Could you check a few things on this model? Use its own coordinates, in mm. A direction names the side the tool comes from. Coordinates: 2 decimals unless noted, no trailing zeros. Loops run counter-clockwise (first coordinate to the right, second up) from the corner with the lowest first, then second, coordinate; pieces in that order, holes last.
1) Thinking about a two-plate mould opening in Z: for faces 5 (the face through (6.4, 145, -75)), 6 (the face through (3, 102, -52.4)), 7 (the face through (3, -3, -2.7)), which applies, released by +Z, released by -Z, zero draft, split by the parting line, or undercut?
2) Imagine slicing it at A-A on y = 20. Please give me the cut outline in (x, z), plus the area to 3 significant figures.
3) Imagine slicing it at C-C on y = 118. Please give me the cut outline in (x, z), plus the area to 3 significant figures.
4) Imagine slicing it at D-D on z = -10. Please give me the cut outline in (x, y), plus the area to 3 significant figures.
5) Will these pins go through, and if not, where does the flat tip stop? P1, Ø1.9, axis at x = 3.5, z = -75.5, coming from the -Y side; P2, Ø3.5, axis at y = 264, z = -76.2, coming from the -X side; P3, Ø1.9, axis at x = 4.5, y = 74.5, coming from the +Z side.
6) For faces 1 (the face through (3, 0, -49)), 2 (the face through (3, 291, -43.7)), 3 (the face through (3, 75, -52.4)), 4 (the face through (3, -6.4, -117)), which set-ups out of +Z, -Z, +X, -X, +Y, -Y let a thin tool reach every point of the face, with its end or its side?
7) If I drill on line 1 along Z through (x, y) = (3.5, 288) (3 decimals); line 2 along Z through (x, y) = (3.75, 20); line 3 along Z through (x, y) = (6, 107.5), over which ranges is the centre line in solid material (lowest first)?
8) Imagine slicing it at B-B on x = 4.5. Give the number of separate pieces and of enclosed holes in the cut face, plus the area to 3 significant figures.
Autodesk Inventor part; units mm, degrees
ref_plane "YZ Plane" through (0, 0, 0) normal (1, 0, 0) x (0, 1, 0)
ref_plane "XZ Plane" through (0, 0, 0) normal (0, 1, 0) x (-1, 0, 0)
ref_plane "XY Plane" through (0, 0, 0) normal (0, 0, 1) x (1, 0, 0)
sketch "Sketch1" plane through (0, 0, 0) normal (1, 0, 0) x (0, 1, 0)
  line L0 (0, 0) -> (0, -152.4) construction
  line L1 (390, -43.7) -> (0, -43.7) construction
  line L2 (0, -43.7) -> (0, -108.7) construction
  line L3 (0, -108.7) -> (390, -108.7) construction
  line L4 (390, -108.7) -> (390, -43.7) construction
  line L5 (0, 0) -> (0, -152.4)
  line L6 (0, 0) -> (195, -43.7)
  line L7 (0, -152.4) -> (195, -108.7)
  line L8 (195, -43.7) -> (390, -43.7)
  line L9 (390, -43.7) -> (390, -108.7)
  line L10 (390, -108.7) -> (195, -108.7)
  circle A0 centre (384, -76.2) radius 2.875
  line L11 (390, -66.2) -> (366, -66.2)
  line L12 (366, -86.2) -> (390, -86.2)
  line L13 (390, -86.2) -> (390, -66.2)
  circle A1 centre (372, -76.2) radius 2.875
  line L14 (0, -2.7) -> (-6.4, -2.7)
  line L15 (-6.4, -2.7) -> (-6.4, -14.7)
  line L16 (-6.4, -14.7) -> (0, -14.7)
  line L17 (0, -14.7) -> (0, -2.7)
  line L18 (-6.4, -29.7) -> (-6.4, -41.7)
  line L19 (-6.4, -41.7) -> (0, -41.7)
  line L20 (0, -29.7) -> (-6.4, -29.7)
  line L21 (-6.4, -56.7) -> (-6.4, -68.7)
  line L22 (-6.4, -68.7) -> (0, -68.7)
  line L23 (0, -56.7) -> (-6.4, -56.7)
  line L24 (-6.4, -83.7) -> (-6.4, -95.7)
  line L25 (-6.4, -95.7) -> (0, -95.7)
  line L26 (0, -83.7) -> (-6.4, -83.7)
  line L27 (-6.4, -110.7) -> (-6.4, -122.7)
  line L28 (-6.4, -122.7) -> (0, -122.7)
  line L29 (0, -110.7) -> (-6.4, -110.7)
  line L30 (-6.4, -137.7) -> (-6.4, -149.7)
  line L31 (-6.4, -149.7) -> (0, -149.7)
  line L32 (0, -137.7) -> (-6.4, -137.7)
  line L33 (27, -46) -> (15, -46)
  line L34 (15, -46) -> (15, -52.4)
  line L35 (15, -52.4) -> (27, -52.4)
  line L36 (27, -52.4) -> (27, -46)
  line L37 (27, -49.2) -> (15, -49.2) construction
  line L38 (42, -52.4) -> (54, -52.4)
  line L39 (54, -46) -> (42, -46)
  line L40 (42, -46) -> (42, -52.4)
  line L41 (54, -52.4) -> (54, -46)
  line L42 (69, -52.4) -> (81, -52.4)
  line L43 (81, -46) -> (69, -46)
  line L44 (69, -46) -> (69, -52.4)
  line L45 (81, -52.4) -> (81, -46)
  line L46 (96, -52.4) -> (108, -52.4)
  line L47 (108, -46) -> (96, -46)
  line L48 (96, -46) -> (96, -52.4)
  line L49 (108, -52.4) -> (108, -46)
  line L50 (96, -106.4) -> (108, -106.4)
  line L51 (108, -100) -> (96, -100)
  line L52 (96, -100) -> (96, -106.4)
  line L53 (108, -106.4) -> (108, -100)
  line L54 (69, -106.4) -> (81, -106.4)
  line L55 (69, -100) -> (69, -106.4)
  line L56 (81, -100) -> (69, -100)
  line L57 (81, -106.4) -> (81, -100)
  line L58 (42, -106.4) -> (54, -106.4)
  line L59 (54, -100) -> (42, -100)
  line L60 (54, -106.4) -> (54, -100)
  line L61 (42, -100) -> (42, -106.4)
  line L62 (15, -106.4) -> (27, -106.4)
  line L63 (15, -100) -> (15, -106.4)
  line L64 (27, -100) -> (15, -100)
  line L65 (27, -106.4) -> (27, -100)
  line L66 (366, -66.2) -> (366, -86.2)
  circle A2 centre (360, -76.2) radius 2.875
  circle A3 centre (348, -76.2) radius 2.875
  line L67 (366, -66.2) -> (342, -66.2)
  line L68 (342, -86.2) -> (366, -86.2)
  line L69 (342, -66.2) -> (342, -86.2)
  circle A4 centre (336, -76.2) radius 2.875
  circle A5 centre (324, -76.2) radius 2.875
  line L70 (342, -66.2) -> (318, -66.2)
  line L71 (318, -86.2) -> (342, -86.2)
  line L72 (318, -66.2) -> (318, -86.2)
  circle A6 centre (312, -76.2) radius 2.875
  circle A7 centre (300, -76.2) radius 2.875
  line L73 (318, -66.2) -> (294, -66.2)
  line L74 (294, -86.2) -> (318, -86.2)
  line L75 (294, -66.2) -> (294, -86.2)
  circle A8 centre (288, -76.2) radius 2.875
  circle A9 centre (276, -76.2) radius 2.875
  line L76 (294, -66.2) -> (270, -66.2)
  line L77 (270, -86.2) -> (294, -86.2)
  line L78 (270, -66.2) -> (270, -86.2)
  circle A10 centre (264, -76.2) radius 2.875
  circle A11 centre (252, -76.2) radius 2.875
  line L79 (270, -66.2) -> (246, -66.2)
  line L80 (246, -86.2) -> (270, -86.2)
  line L81 (246, -66.2) -> (246, -86.2)
  circle A12 centre (240, -76.2) radius 2.875
  circle A13 centre (228, -76.2) radius 2.875
  line L82 (246, -66.2) -> (222, -66.2)
  line L83 (222, -86.2) -> (246, -86.2)
  line L84 (222, -66.2) -> (222, -86.2)
  circle A14 centre (216, -76.2) radius 2.875
  circle A15 centre (204, -76.2) radius 2.875
  line L85 (222, -66.2) -> (198, -66.2)
  line L86 (198, -86.2) -> (222, -86.2)
  line L87 (198, -66.2) -> (198, -86.2)
  circle A16 centre (192, -76.2) radius 2.875
  circle A17 centre (180, -76.2) radius 2.875
  line L88 (198, -66.2) -> (174, -66.2)
  line L89 (174, -86.2) -> (198, -86.2)
  line L90 (174, -66.2) -> (174, -86.2)
  circle A18 centre (168, -76.2) radius 2.875
  circle A19 centre (156, -76.2) radius 2.875
  line L91 (174, -66.2) -> (150, -66.2)
  line L92 (150, -86.2) -> (174, -86.2)
  line L93 (150, -66.2) -> (150, -86.2)
  point P0 (390, -86.2)
  point P1 (390, -66.2)
  point P2 (0, -8.7)
  point P3 (0, -149.7)
  point P4 (0, -122.7)
  point P5 (0, -95.7)
  point P6 (0, -68.7)
  point P7 (0, -41.7)
  point P8 (117.4088, -76.2)
  point P9 (42, -49.2)
  point P10 (54, -49.2)
  point P11 (69, -49.2)
  point P12 (81, -49.2)
  point P13 (96, -49.2)
  point P14 (108, -49.2)
  point P15 (108, -103.2)
  point P16 (96, -103.2)
  point P17 (69, -103.2)
  point P18 (81, -103.2)
  point P19 (54, -103.2)
  point P20 (42, -103.2)
  point P21 (15, -103.2)
  point P22 (27, -103.2)
  dimension "d0" = 152.4
  dimension "d1" = 65
  dimension "d2" = 390
  dimension "d4" = 5.75
  dimension "d5" = 20
  dimension "d8" = 5.75
  dimension "d11" = 0
  dimension "d21" = 12
  dimension "d22" = 6.4
  dimension "d23" = 2.7
  dimension "d26" = 27
  dimension "d39" = 12
  dimension "d40" = 6.4
  dimension "d41" = 46
  dimension "d42" = 15
  dimension "d45" = 27
  dimension "d52" = 54
  dimension "d57" = 12
  dimension "d58" = 6
  dimension "d59" = 6
  dimension "d62" = 24
extrude "Extrusion1" add sketch "Sketch1" along normal blind 6.4
properties part number "mdf_vertical_r1"
Filled in:
1. face 5: zero draft
1. face 6: undercut
1. face 7: released by +Z
2. outline: (0, -147.92) - (6.4, -147.92) - (6.4, -106.4) - (0, -106.4) - close; (0, -100) - (6.4, -100) - (6.4, -52.4) - (0, -52.4) - close; (0, -46) - (6.4, -46) - (6.4, -4.48) - (0, -4.48) - close
2. area: 836 mm2
3. outline: (0, -125.96) - (6.4, -125.96) - (6.4, -26.44) - (0, -26.44) - close
3. area: 637 mm2
4. outline: (0, -6.4) - (6.4, -6.4) - (6.4, 44.62) - (0, 44.62) - close
4. area: 327 mm2
5. P1: stops at y = 0
5. P2: passes through
5. P3: stops at z = -16.48
6. face 1: +X, -X, -Y
6. face 2: +Z, +X, -X, +Y
6. face 3: +X, -X
6. face 4: +Z, -Z, +X, -X, -Y
7. line 1: z = -108.7 to -79.075, -73.325 to -43.7
7. line 2: z = -147.92 to -106.4, -100 to -52.4, -46 to -4.48
7. line 3: z = -128.31 to -106.4, -100 to -52.4, -46 to -24.09
8. separate pieces: 1
8. enclosed holes: 28
8. area: 33,200 mm2
